Autodesk Inventor part; units mm, degrees
ref_plane "YZ Plane" through (0, 0, 0) normal (1, 0, 0) x (0, 1, 0)
ref_plane "XZ Plane" through (0, 0, 0) normal (0, 1, 0) x (-1, 0, 0)
ref_plane "XY Plane" through (0, 0, 0) normal (0, 0, 1) x (1, 0, 0)
sketch "Skizze1" plane through (0, 0, 0) normal (0, 1, 0) x (-1, 0, 0)
  line L0 (48.5149, -32.0545) -> (13.5149, -32.0545)
  line L1 (13.5149, -32.0545) -> (13.5149, -102.0545)
  line L2 (13.5149, -102.0545) -> (48.5149, -102.0545)
  line L3 (48.5149, -102.0545) -> (48.5149, -32.0545)
  point P0 (0, 0)
  dimension "d0" = 70
  dimension "d1" = 35
extrude "Extrusion1" add sketch "Skizze1" along normal blind 40
sketch "Skizze2" plane through (-13.5149, 0, -32.0545) normal (1, 0, 0) x (0, 0, -1)
  circle A0 centre (55, 15) radius 1.5
  circle A1 centre (55, 15) radius 2.5
  line L0 (0, 0) -> (70, 0)
  line L1 (70, 0) -> (70, 40)
  point P0 (-32.0545, 0)
  dimension "d4" = 3
  dimension "d5" = 5
  dimension "d10" = 15
  dimension "d11" = 15
extrude "Extrusion2" add sketch "Skizze2" along normal blind 40 contours A0
extrude "Extrusion3" add sketch "Skizze2" along normal blind 10
properties part number "Motor_rechts"
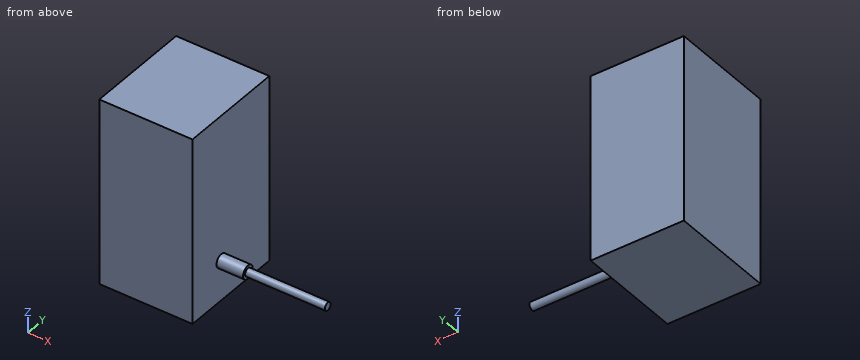
Here's how the part is built. I have some questions about the finished solid (model axes, mm). Round coordinates to 2 decimals unless told otherwise and drop trailing zeros. Order: outer loops, then holes, each group sorted by start corner. A loop starts at its lowest first (then second) coordinate and runs counter-clockwise, first axis right, second up. Notation, with made-up numbers: M 18,-7.75 L 61,-7.75 A28 ccw 61,16.25 Z; hole C 78.25,-25.5 d7. An arc over 180 degrees is marked long. Answer as CSV lines item,"result".
Item 1: Imagine slicing it at B-B on z = -74. List the corners of the cut face in (x, y) for me, and give its area (3 significant figures).
From the geometry:
outline,"M -48.51,0 L -13.51,0 L -13.51,40 L -48.51,40 Z"
area,"1,400 mm2"
Item 2: Please list where these lines run through material, in increasing order: L1, parallel to X at y = 13, z = -59.5; L2, parallel to Z at x = -7, y = 16.5. Write a range as [from, to].
From the geometry:
L1,"[-48.51, -13.51]"
L2,"[-89.05, -85.05]"
Item 3: Imagine slicing it at A-A on y = 15. List the corners of the cut face in (x, z) for me, and give its area (3 significant figures).
From the geometry:
outline,"M -48.51,-102.05 L -13.51,-102.05 L -13.51,-89.55 L -3.51,-89.55 L -3.51,-88.55 L 26.49,-88.55 L 26.49,-85.55 L -3.51,-85.55 L -3.51,-84.55 L -13.51,-84.55 L -13.51,-32.05 L -48.51,-32.05 Z"
area,"2,590 mm2"
Item 4: Imagine slicing it at C-C on x = 20. List the corners of the cut face in (y, z) for me.
From the geometry:
outline,"C 15,-87.05 d3"
Item 5: Imagine slicing it at D-D on y = 26.5. List the corners of the cut face in (x, z) for me.
From the geometry:
outline,"M -48.51,-102.05 L -13.51,-102.05 L -13.51,-32.05 L -48.51,-32.05 Z"
Item 6: For pin 1 (12 mm diameter, centred on y = 20.5, z = -75, fed in from +X); pin 2 (2 mm diameter, centred on x = -18, z = -65.5, fed in from -Y), each with a flat end and sliding along its axis, tell me the tip position at first contact or that it passes through.
From the geometry:
pin 1,"x = -13.51"
pin 2,"y = 0"
